Design review of the part built by this model. Coordinates are the model's own, in mm. A direction names the side the tool comes from. Coordinates: 2 decimals unless noted, no trailing zeros. Loops run counter-clockwise (first coordinate to the right, second up) from the corner with the lowest first, then second, coordinate; pieces in that order, holes last. Notation, with made-up numbers: (-38, 89.25) -> (-17, 89.25) arc R20 ccw to (-17, 122.25) -> close; hole circle Ø4 at (87, -30). An arc over 180 degrees is marked (long way). Answer in a Markdown table with one row per item.
```python
from build123d import *

# Parameters (mm, degrees)
F1_DEPTH = 1270
F3_DEPTH = 127
F5_DEPTH = 25.4
F6_R     = 6.35
F7_DEPTH = 25.4


# Not quite as in the source:
# - a feature names something its author has since deleted; it is built from what else it names


with BuildPart() as f1:
    # F0 (on Front) → F1 (new body)
    with BuildSketch(Plane.XZ):
        Polygon((3.175, 50.8), (0, 50.8), (0, 0), (50.8, 0), (50.8, 3.175), (3.175, 3.175), align=None)
    extrude(amount=F1_DEPTH)

    # F2 (on face) → F3 (intersect)
    with BuildSketch(Plane(origin=(0, 0, 0), x_dir=(1, 0, 0), z_dir=(0, 0, -1))):
        Polygon((0, 1022.35), (0, 0), (50.8, 50.8), (50.8, 971.55), align=None)
    extrude(amount=-F3_DEPTH, mode=Mode.INTERSECT)

    # F4 (on face) → F5 (cut)
    with BuildSketch(Plane.YZ.offset(3.175)):
        with BuildLine():
            ThreePointArc((-885.825155029, 28.3765627422), (-892.1701940961, 34.7265608044), (-898.5251472776, 28.3864846051))
            Line((-898.5251472776, 28.3864846051), (-885.8251627805, 28.3666408793))
            ThreePointArc((-885.8251627805, 28.3666408793), (-885.8251569669, 28.3716018093), (-885.825155029, 28.3765627422))
        make_face()
        with BuildLine():
            ThreePointArc((-123.825155029, 28.3765627422), (-130.7681849335, 34.6988104068), (-136.4143882675, 27.1956865442))
            Line((-136.4143882675, 27.1956865442), (-123.9396424845, 27.1761947539))
            ThreePointArc((-123.9396424845, 27.1761947539), (-123.8538416901, 27.7736550617), (-123.825155029, 28.3765627422))
        make_face()
        with BuildLine():
            Line((-123.9396424845, 27.1761947539), (-136.4143882675, 27.1956865442))
            ThreePointArc((-136.4143882675, 27.1956865442), (-130.1850768919, 22.0265704937), (-123.9396424845, 27.1761947539))
        make_face()
        with BuildLine():
            ThreePointArc((-250.825155029, 28.3765627422), (-257.6678327049, 34.7074211917), (-263.4487042283, 27.3941776629))
            Line((-263.4487042283, 27.3941776629), (-250.9047064081, 27.3745776663))
            ThreePointArc((-250.9047064081, 27.3745776663), (-250.8450741155, 27.8739937135), (-250.825155029, 28.3765627422))
        make_face()
        with BuildLine():
            Line((-250.9047064081, 27.3745776663), (-263.4487042283, 27.3941776629))
            ThreePointArc((-263.4487042283, 27.3941776629), (-257.1850768919, 22.0265704937), (-250.9047064081, 27.3745776663))
        make_face()
        with BuildLine():
            ThreePointArc((-377.825155029, 28.3765627422), (-384.567858719, 34.7144081026), (-390.4765830013, 27.5926587234))
            Line((-390.4765830013, 27.5926587234), (-377.8762075195, 27.5729706367))
            ThreePointArc((-377.8762075195, 27.5729706367), (-377.837931004, 27.9739566603), (-377.825155029, 28.3765627422))
        make_face()
        with BuildLine():
            Line((-377.8762075195, 27.5729706367), (-390.4765830013, 27.5926587234))
            ThreePointArc((-390.4765830013, 27.5926587234), (-384.1850768919, 22.0265704937), (-377.8762075195, 27.5729706367))
        make_face()
        with BuildLine():
            ThreePointArc((-504.825155029, 28.3765627422), (-511.4681836347, 34.7197980552), (-517.498110694, 27.7911298605))
            Line((-517.498110694, 27.7911298605), (-504.8540597111, 27.7713735308))
            ThreePointArc((-504.8540597111, 27.7713735308), (-504.8323853158, 28.0736232011), (-504.825155029, 28.3765627422))
        make_face()
        with BuildLine():
            Line((-504.8540597111, 27.7713735308), (-517.498110694, 27.7911298605))
            ThreePointArc((-517.498110694, 27.7911298605), (-511.1850768919, 22.0265704937), (-504.8540597111, 27.7713735308))
        make_face()
        with BuildLine():
            ThreePointArc((-631.825155029, 28.3765627422), (-638.3687307774, 34.7236115391), (-644.5133529596, 27.9895911765))
            Line((-644.5133529596, 27.9895911765), (-631.8381973298, 27.9697862458))
            ThreePointArc((-631.8381973298, 27.9697862458), (-631.8284164417, 28.1730699785), (-631.825155029, 28.3765627422))
        make_face()
        with BuildLine():
            Line((-631.8381973298, 27.9697862458), (-644.5133529596, 27.9895911765))
            ThreePointArc((-644.5133529596, 27.9895911765), (-638.1850768919, 22.0265704937), (-631.8381973298, 27.9697862458))
        make_face()
        with BuildLine():
            ThreePointArc((-758.825155029, 28.3765627422), (-765.2694254172, 34.7258629473), (-771.5223560035, 28.1880427438))
            Line((-771.5223560035, 28.1880427438), (-758.8285741702, 28.1682087096))
            ThreePointArc((-758.8285741702, 28.1682087096), (-758.8260098719, 28.2723716996), (-758.825155029, 28.3765627422))
        make_face()
        with BuildLine():
            Line((-758.8285741702, 28.1682087096), (-771.5223560035, 28.1880427438))
            ThreePointArc((-771.5223560035, 28.1880427438), (-765.1850768919, 22.0265704937), (-758.8285741702, 28.1682087096))
        make_face()
        with BuildLine():
            Line((-885.8251627805, 28.3666408793), (-898.5251472776, 28.3864846051))
            ThreePointArc((-898.5251472776, 28.3864846051), (-892.1850768919, 22.0265704937), (-885.8251627805, 28.3666408793))
        make_face()
    extrude(amount=-F5_DEPTH, mode=Mode.SUBTRACT)

    # F6 (on face) → F7 (cut)
    with BuildSketch(Plane.XY.offset(3.175)):
        with BuildLine():
            ThreePointArc((33.3375, -828.675), (22.4973719395, -824.1848719395), (26.9875, -835.025))
            ThreePointArc((26.9875, -835.025), (31.4776280605, -833.1651280605), (33.3375, -828.675))
        make_face()
        with Locations((26.9875, -701.675)):
            Circle(F6_R)
        with Locations((26.9875, -574.675)):
            Circle(F6_R)
        with Locations((26.9875, -447.675)):
            Circle(F6_R)
        with Locations((26.9875, -193.675)):
            Circle(F6_R)
        with Locations((26.9875, -320.675)):
            Circle(F6_R)
    extrude(amount=-F7_DEPTH, mode=Mode.SUBTRACT)


solid = f1.part
```
(1) Tool access review of faces 1 (the flat face through (0, -504, 26)), 2 (the flat face through (27, -504, 3.175)): name each direction out of +Z, -Z, +X, -X, +Y, -Y from which nothing blocks a thin tool from reaching the whole face with its end or side.
Evaluation:
| item | result |
|---|---|
| face 1 | +Z, -Z, -X, +Y, -Y |
| face 2 | +Z, +X, +Y, -Y |
(2) Take a section at A-A on y = -861.5. Give the boundary of the cut face in (x, z) (3 decimals).
Evaluation:
| item | result |
|---|---|
| outline | (0, 0) -> (50.8, 0) -> (50.8, 3.175) -> (3.175, 3.175) -> (3.175, 50.8) -> (0, 50.8) -> close |
(3) Take a section at B-B on z = 14. Give the boundary of the cut face in (x, y) (3 decimals).
Evaluation:
| item | result |
|---|---|
| outline | (0, -1022.35) -> (3.175, -1019.175) -> (3.175, -3.175) -> (0, 0) -> close |
(4) For pin 1 (1 mm diameter, centred on x = 17, y = -804.5, fed in from -Z); pin 2 (1.5 mm diameter, centred on y = -835, z = 16, fed in from +X) (3 decimals); pin 3 (6 mm diameter, centred on x = 11, y = -490, fed in from +Z) (3 decimals), all flat-tipped, find the tip position at first contact; note any pin that passes through.
Evaluation:
| item | result |
|---|---|
| pin 1 | stops at z = 0 |
| pin 2 | stops at x = 3.175 |
| pin 3 | stops at z = 3.175 |
(5) To check wall thickness, follow probe 1 along Z at (x, y) = (14, -366.5) (3 decimals). State the ranges of the line that lie inside material, in increasing order.
Evaluation:
| item | result |
|---|---|
| probe 1 | z = 0 to 3.175 |
